The listing builds one solid part. Answer for the finished solid, in the listing's coordinates (mm). A direction names the side the tool comes from. Coordinates: 2 decimals unless noted, no trailing zeros. Order: outer loops, then holes, each group sorted by start corner. A loop starts at its lowest first (then second) coordinate and runs counter-clockwise, first axis right, second up. Notation, with made-up numbers: (-15, 59.25) -> (17, 59.25) arc R16 ccw to (17, 86.25) -> close; hole circle Ø1 at (39, 64.5). An arc over 180 degrees is marked (long way). Answer in a Markdown table with one row per item.
Autodesk Inventor part; units mm, degrees
ref_plane "YZ Plane" through (0, 0, 0) normal (1, 0, 0) x (0, 1, 0)
ref_plane "XZ Plane" through (0, 0, 0) normal (0, 1, 0) x (-1, 0, 0)
ref_plane "XY Plane" through (0, 0, 0) normal (0, 0, 1) x (1, 0, 0)
sketch "Szkic1" plane through (0, 0, 0) normal (0, 1, 0) x (-1, 0, 0)
  point P0 (0, 0)
sketch "Szkic2" plane through (0, 0, 0) normal (0, 1, 0) x (-1, 0, 0)
  line L0 (50, -14.4) -> (-50, -14.4)
  line L1 (-50, -14.4) -> (-50, 14.4)
  line L2 (-50, 14.4) -> (50, 14.4)
  line L3 (50, 14.4) -> (50, -14.4)
  line L4 (50, -14.4) -> (-50, 14.4) construction
  line L5 (-50, -14.4) -> (50, 14.4) construction
  point P0 (0, 0)
  dimension "d0" = 100
  dimension "d1" = 28.8
extrude "Wyciągnięcie proste1" add sketch "Szkic2" along normal blind 4
sketch "Szkic3" plane through (0, 4, 0) normal (0, 1, 0) x (1, 0, 0)
  line L0 (-0.6, 14.4) -> (0.6, 14.4)
  line L1 (0.6, 14.4) -> (0.6, -14.4)
  line L2 (0.6, -14.4) -> (-0.6, -14.4)
  line L3 (-0.6, -14.4) -> (-0.6, 14.4)
  line L4 (-0.6, 14.4) -> (0.6, -14.4) construction
  line L5 (0.6, 14.4) -> (-0.6, -14.4) construction
  point P0 (0, 0)
  dimension "d4" = 1.2
  dimension "d5" = 28.8
extrude "Wyciągnięcie proste2" add sketch "Szkic3" along normal blind 22
sketch "Szkic4" plane through (-50, 0, 14.4) normal (0, 0, 1) x (1, 0, 0)
  line L0 (0, 0) -> (0, 4)
  line L1 (50.6, 26) -> (49.4, 26)
  line L2 (0, 4) -> (49.4, 26)
  line L3 (0, 4) -> (49.4, 4)
  line L4 (49.4, 26) -> (49.4, 4)
  line L5 (49.4, 4) -> (0, 4)
  point P0 (50, 0)
extrude "Wyciągnięcie proste3" add sketch "Szkic4" against normal blind 1.2
mirror "Odbij1" about plane through (0, 0, 0) normal (1, 0, 0) of "Wyciągnięcie proste3"
mirror "Odbij2" about plane through (0, 0, 0) normal (0, 0, 1) of "Wyciągnięcie proste3", "Odbij1"
sketch "Szkic5" plane through (-50, 0, 14.4) normal (0, 0, 1) x (1, 0, 0)
  point P0 (50, 0)
sketch "Szkic6" plane through (-50, 0, 14.4) normal (0, 0, 1) x (1, 0, 0)
  line L0 (50, 0) -> (50, -3)
  circle A0 centre (50, -3) radius 11.6
  dimension "d10" = 3
  dimension "d11" = 23.2
extrude "Wyciągnięcie proste4" add sketch "Szkic6" against normal blind 8
sketch "Szkic7" plane through (-50, 0, 14.4) normal (0, 0, 1) x (1, 0, 0)
  line L0 (50, 0) -> (50, -4)
  circle A0 centre (50, -4) radius 11
  dimension "d14" = 4
  dimension "d15" = 22
extrude "Wyciągnięcie proste5" cut sketch "Szkic7" against normal blind 6.8
mirror "Odbij3" about plane through (0, 0, 0) normal (0, 0, 1) of "Wyciągnięcie proste4", "Wyciągnięcie proste5"
sketch "Szkic8" plane through (0, 0, 0) normal (0, -1, 0) x (1, 0, 0)
  line L0 (50, -14.4) -> (-50, -14.4)
  line L1 (-50, -14.4) -> (-50, 14.4)
  line L2 (-50, 14.4) -> (50, 14.4)
  line L3 (50, 14.4) -> (50, -14.4)
  line L4 (50, -14.4) -> (-50, 14.4) construction
  line L5 (-50, -14.4) -> (50, 14.4) construction
  point P0 (0, 0)
  dimension "d18" = 100
  dimension "d19" = 28.8
extrude "Wyciągnięcie proste6" cut sketch "Szkic8" along normal through all
sketch "Szkic9" plane through (0, 0, 0) normal (0, -1, 0) x (1, 0, 0)
  line L0 (50, 14.4) -> (50, -14.4)
  line L1 (50, 0) -> (43, 0)
  line L2 (36, -14) -> (50, -14)
  line L3 (50, -14) -> (50, 14)
  line L4 (50, 14) -> (36, 14)
  line L5 (36, 14) -> (36, -14)
  line L6 (36, -14) -> (50, 14) construction
  line L7 (50, -14) -> (36, 14) construction
  point P0 (0, 0)
  point P1 (50, -14)
  point P2 (50, 14)
  dimension "d22" = 7
  dimension "d23" = 14
  dimension "d24" = 28
extrude "Wyciągnięcie proste7" cut sketch "Szkic9" against normal blind 2.8
mirror "Odbij4" about plane through (0, 0, 0) normal (1, 0, 0) of "Wyciągnięcie proste7"
sketch "Szkic10" plane through (0, 0, 0) normal (0, -1, 0) x (1, 0, 0)
  line L0 (50, -14.4) -> (-50, -14.4)
  line L1 (-50, -14.4) -> (-50, 14.4)
  line L2 (-50, 14.4) -> (50, 14.4)
  line L3 (50, 14.4) -> (50, -14.4)
  line L4 (50, -14.4) -> (-50, 14.4) construction
  line L5 (-50, -14.4) -> (50, 14.4) construction
  point P0 (0, 0)
  dimension "d27" = 100
  dimension "d28" = 28.8
sketch "Szkic11" plane through (0, 0, 0) normal (0, -1, 0) x (1, 0, 0)
  line L0 (-50, 14.4) -> (50, 14.4)
  line L1 (50, 14.4) -> (50, -14.4)
  line L2 (50, -14.4) -> (-50, -14.4)
  line L3 (-50, -14.4) -> (-50, 14.4)
  line L4 (-50, 14.4) -> (50, -14.4) construction
  line L5 (50, 14.4) -> (-50, -14.4) construction
  point P0 (0, 0)
  dimension "d29" = 100
  dimension "d30" = 28.8
extrude "Wyciągnięcie proste8" cut sketch "Szkic11" against normal blind 0.4
properties part number "kolyska_v2"
(1) A cutting plane is placed at B-B, the plane y = 12.75. Determine the outline of the cut face in (x, z), then the cut area to 3 significant figures.
Check values:
| item | result |
|---|---|
| outline | (-30.35, -14.4) -> (30.35, -14.4) -> (30.35, -13.2) -> (0.6, -13.2) -> (0.6, 13.2) -> (30.35, 13.2) -> (30.35, 14.4) -> (-30.35, 14.4) -> (-30.35, 13.2) -> (-0.6, 13.2) -> (-0.6, -13.2) -> (-30.35, -13.2) -> close |
| area | 177 mm² |
(2) A cutting plane is placed at C-C, the plane x = -13. Determine the outline of the cut face in (y, z), then the cut area to 3 significant figures.
Check values:
| item | result |
|---|---|
| outline | (0.4, -14.4) -> (20.48, -14.4) -> (20.48, -13.2) -> (4, -13.2) -> (4, 13.2) -> (20.48, 13.2) -> (20.48, 14.4) -> (0.4, 14.4) -> close |
| area | 143 mm² |
(3) For a pull along X with two mould halves and no side action, classify faces 1 (the cylindrical face through (0, 7, 11)), 2 (the flat face through (43, 2.8, 0)), 3 (the flat face through (0.6, 15, 0)) as released by +X, released by -X, zero draft, split by the parting line, or undercut.
Check values:
| item | result |
|---|---|
| face 1 | undercut |
| face 2 | zero draft |
| face 3 | released by +X |
(4) Which of the six approach directions +Z, -Z, +X, -X, +Y, -Y give full straight-line access (tool end or side, diameter ignored) to faces 4 (the flat face through (-43, 2, -14)), 5 (the flat face through (-4, 6, -6.4)), 6 (the cylindrical face through (0, 7, -11)), 7 (the flat face through (43, 2, 14))?
Check values:
| item | result |
|---|---|
| face 4 | -X, -Y |
| face 5 | -X, +Y |
| face 6 | -Z, -Y |
| face 7 | +X, -Y |
(5) A cutting plane is placed at D-D, the plane z = 0.75. Determine the outline of the cut face in (x, y).
Check values:
| item | result |
|---|---|
| outline | (-50, 2.8) -> (-36, 2.8) -> (-36, 0.4) -> (36, 0.4) -> (36, 2.8) -> (50, 2.8) -> (50, 4) -> (0.6, 4) -> (0.6, 26) -> (-0.6, 26) -> (-0.6, 4) -> (-50, 4) -> close |
(6) Flat-ended cylindrical pins translate along their axes: pin 1 (3 mm diameter, centred on y = 21.5, z = -7.5, fed in from +X); pin 2 (3 mm diameter, centred on y = 8.5, z = 8, fed in from +X); pin 3 (4 mm diameter, centred on x = -45, z = 6.5, fed in from -Y). Find the tip coordinate at first contact, or state that the pin passes through.
Check values:
| item | result |
|---|---|
| pin 1 | x = 0.6 |
| pin 2 | x = 5.88 |
| pin 3 | y = 2.8 |
(7) A cutting plane is placed at A-A, the plane z = 8.75. Determine the outline of the cut face in (x, y), then the cut area to 3 significant figures.
Check values:
| item | result |
|---|---|
| outline | (-50, 2.8) -> (-36, 2.8) -> (-36, 0.4) -> (-10.08, 0.4) arc R11 cw to (10.08, 0.4) -> (36, 0.4) -> (36, 2.8) -> (50, 2.8) -> (50, 4) -> (9.25, 4) arc R11.6 ccw to (0.6, 8.58) -> (0.6, 26) -> (-0.6, 26) -> (-0.6, 8.58) arc R11.6 ccw to (-9.25, 4) -> (-50, 4) -> close |
| area | 277 mm² |
(8) Find the intervals of material crossed by line 1 along Z through (x, y) = (-11, 12.5); line 2 along X through (y, z) = (9.25, 6); line 3 along Y through (x, z) = (-34, 1), in increasing order. Write a range as from..to.
Check values:
| item | result |
|---|---|
| line 1 | -14.4..-13.2, 13.2..14.4 |
| line 2 | -0.6..0.6 |
| line 3 | 0.4..4 |
